```python
from build123d import *

# Parameters (mm, degrees)
SKETCH1_R               = 22.567960526
BOSS_EXTRUDE1_DEPTH     = 5
SKETCH2_W               = 45.135921052
SKETCH2_H               = 25.616013259
BOSS_EXTRUDE2_DEPTH     = 5
SKETCH3_R               = 1.5
SKETCH3_R_2             = 3.55
CUT_EXTRUDE1_DEPTH      = 1
CUT_EXTRUDE1_DEPTH_BACK = 6
SKETCH4_W               = 35.135921052
SKETCH4_H               = 3.066013259
CUT_EXTRUDE2_DEPTH      = 2.5
BOSS_EXTRUDE3_DEPTH     = 4


with BuildPart() as part:
    # Sketch1 → Boss-Extrude1 (new body)
    with BuildSketch(Plane(origin=(0, 0, 0), x_dir=(0, 0, -1), z_dir=(1, 0, 0))):
        Circle(SKETCH1_R)
    extrude(amount=BOSS_EXTRUDE1_DEPTH)

    # Sketch2 → Boss-Extrude2 (add)
    with BuildSketch(Plane(origin=(5, 0, 0), x_dir=(0, 0, -1), z_dir=(1, 0, 0))):
        with Locations((0, -12.80800663)):
            Rectangle(SKETCH2_W, SKETCH2_H)
    extrude(amount=-BOSS_EXTRUDE2_DEPTH)

    # Sketch3 → Cut-Extrude1 (cut, two sides)
    with BuildSketch(Plane(origin=(5, 0, 0), x_dir=(0, 0, -1), z_dir=(1, 0, 0))) as cut_extrude1_sk:
        with Locations((-3, 13.371154887)):
            Circle(SKETCH3_R)
        with Locations((3, 13.371154887)):
            Circle(SKETCH3_R)
        Circle(SKETCH3_R_2)
    extrude(amount=CUT_EXTRUDE1_DEPTH, mode=Mode.SUBTRACT)
    extrude(cut_extrude1_sk.sketch, amount=-CUT_EXTRUDE1_DEPTH_BACK, mode=Mode.SUBTRACT)

    # Sketch4 → Cut-Extrude2 (cut)
    with BuildSketch(Plane(origin=(5, 0, 0), x_dir=(0, 0, -1), z_dir=(1, 0, 0))):
        with Locations((0, -22.08300663)):
            Rectangle(SKETCH4_W, SKETCH4_H)
    extrude(amount=-CUT_EXTRUDE2_DEPTH, mode=Mode.SUBTRACT)

    # Sketch5 → Boss-Extrude3 (add)
    with BuildSketch(Plane(origin=(5, 0, 0), x_dir=(0, 0, -1), z_dir=(1, 0, 0))):
        with BuildLine():
            Line((-11.283980263, 19.544427127), (-9.375, 16.237976321))
            ThreePointArc((-9.375, 16.237976321), (-7.175314357, 17.322741235), (-4.852857096, 18.111109243))
            Line((-4.852857096, 18.111109243), (-5.841017993, 21.798975919))
            ThreePointArc((-5.841017993, 21.798975919), (-8.636384596, 20.850076821), (-11.283980263, 19.544427127))
        make_face()
        with BuildLine():
            Line((5.841017993, 21.798975919), (4.852857096, 18.111109243))
            ThreePointArc((4.852857096, 18.111109243), (7.175314357, 17.322741235), (9.375, 16.237976321))
            Line((9.375, 16.237976321), (11.283980263, 19.544427127))
            ThreePointArc((11.283980263, 19.544427127), (8.636384596, 20.850076821), (5.841017993, 21.798975919))
        make_face()
        with BuildLine():
            Line((-5.506355904, -20.55), (-4.852857096, -18.111109243))
            ThreePointArc((-4.852857096, -18.111109243), (-7.175314357, -17.322741235), (-9.375, -16.237976321))
            Line((-9.375, -16.237976321), (-11.283980263, -19.544427127))
            ThreePointArc((-11.283980263, -19.544427127), (-10.318214034, -20.071056312), (-9.327933443, -20.55))
            Line((-9.327933443, -20.55), (-5.506355904, -20.55))
        make_face()
        with BuildLine():
            Line((11.283980263, -19.544427127), (9.375, -16.237976321))
            ThreePointArc((9.375, -16.237976321), (7.175314357, -17.322741235), (4.852857096, -18.111109243))
            Line((4.852857096, -18.111109243), (5.506355904, -20.55))
            Line((5.506355904, -20.55), (9.327933443, -20.55))
            ThreePointArc((9.327933443, -20.55), (10.318214034, -20.071056312), (11.283980263, -19.544427127))
        make_face()
    extrude(amount=BOSS_EXTRUDE3_DEPTH)


solid = part.part
```
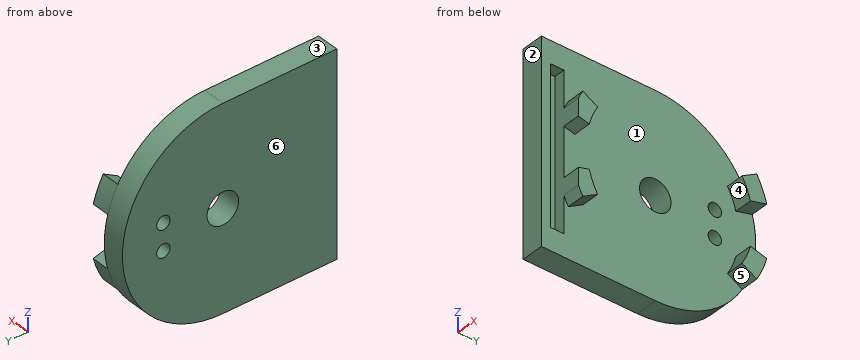
CAD build for the part. Positions are in the model's coordinates, mm. Face numbers are marked on the shaded views. A direction names the side the tool comes from. Round coordinates to 2 decimals unless told otherwise and drop trailing zeros. Write each loop counter-clockwise with the first axis right and the second up, starting at its lowest first coordinate (ties: lowest second). Pieces come first, ordered by that corner, then holes. Notation, with made-up numbers: (34.5, 86) -> (70.5, 86) arc R21 cw to (70.5, 116) -> close; hole circle Ø4 at (-37, 61.25). An arc over 180 degrees is marked (long way). Answer in a Markdown table with one row per item. Add a question column.
Item 1: Which spindle directions (+Z, -Z, +X, -X, +Y, -Y) get a long thin tool onto all of the face, cutting with end or side? Do the marked faces 1 and 2. Say none if no direction does.
Item 2: Saw through at D-D, the plane y = -10.5. Write the cut outline in (x, z), then the cut area to 3 significant figures.
Item 3: Drop flat-ended pins along their axis: pin 1 Ø1.2 at (x, z) = (3, -8) entering from +Y; pin 2 Ø1.5 at (y, z) = (3.5, 16.5) entering from +X; pin 3 Ø2.5 at (y, z) = (-22, 3.5) entering from +X. Give the stop position or say it passes through.
Item 4: Saw through at A-A, the plane z = 0. Write the cut outline in (x, y), then the cut area to 3 significant figures.
Item 5: Saw through at B-B, the plane x = 3.75. Write the cut outline in (y, z).
Item 6: Drill centre lines: line 1 (Y direction, x = 3.15, z = 0); line 2 (Y direction, x = 2.05, z = -3); line 3 (X direction, y = -18, z = -4.5). Where is each one in solid material? Low to high. Write a range as from..to.
Item 7: Mould opens along Z. For the marked faces 3, 4, 5 and 6 say: pulls with the +Z half, pulls with the -Z half, needs draft (parallel to the pull), parting line crosses it, or undercut.
Item 8: Saw through at C-C, the plane z = -7. Write the cut outline in (x, y).
Findings below:
| question | item | result |
|---|---|---|
| 1 | face 1 | +X |
| 1 | face 2 | +Z, -Z, +X, -X, -Y |
| 2 | outline | (0, -22.57) -> (5, -22.57) -> (5, 22.57) -> (0, 22.57) -> close |
| 2 | area | 226 mm^2 |
| 3 | pin 1 | stops at y = 21.32 |
| 3 | pin 2 | stops at x = 5 |
| 3 | pin 3 | stops at x = 2.5 |
| 4 | outline | (0, -25.62) -> (5, -25.62) -> (5, -23.62) -> (2.5, -23.62) -> (2.5, -20.55) -> (5, -20.55) -> (5, -3.55) -> (0, -3.55) -> close; (0, 3.55) -> (5, 3.55) -> (5, 22.57) -> (0, 22.57) -> close |
| 4 | area | 198 mm^2 |
| 5 | outline | (-25.62, -22.57) -> (0, -22.57) arc R22.57 ccw to (0, 22.57) -> (-25.62, 22.57) -> close; hole (-23.62, -17.57) -> (-20.55, -17.57) -> (-20.55, 17.57) -> (-23.62, 17.57) -> close; hole circle Ø7.1 at (0, 0); hole circle Ø3 at (13.37, -3); hole circle Ø3 at (13.37, 3) |
| 6 | line 1 | y = -25.62..-23.62, -20.55..-3.55, 3.55..22.57 |
| 6 | line 2 | y = -25.62..-1.9, 1.9..11.87, 14.87..22.37 |
| 6 | line 3 | x = 0..5 |
| 7 | face 3 | pulls with the +Z half |
| 7 | face 4 | undercut |
| 7 | face 5 | pulls with the -Z half |
| 7 | face 6 | needs draft |
| 8 | outline | (0, -25.62) -> (5, -25.62) -> (5, -23.62) -> (2.5, -23.62) -> (2.5, -20.55) -> (9, -20.55) -> (9, -17.39) -> (5, -17.39) -> (5, 17.39) -> (9, 17.39) -> (9, 21.45) -> (0, 21.45) -> close |
